For this review, take the finished solid that the model builds, in its own axes (mm). A direction names the side the tool comes from. Give positions to 0.01 mm unless a question says otherwise; leave off trailing zeros. Write each loop counter-clockwise with the first axis right and the second up, starting at its lowest first coordinate (ties: lowest second). Pieces come first, ordered by that corner, then holes. Notation, with made-up numbers: M 31,29.5 L 63,29.5 A25 cw 63,60.5 Z; hole C -20,70.25 d4. An arc over 180 degrees is marked long. One line per item, written item: value. Start each with the question number.
Item 1: Consider section B-B, the plane z = 4. Write out the cut boundary in (x, y) (3 decimals), and give its area (3 significant figures).
Item 2: Clearance check with a flat-ended pin moving along its axis: pin 1 Ø4.5 at (x, y) = (40, 106.825) entering from -Z. State where the tip first meets the part, or that it passes through.
Item 3: Mouldability with a two-part tool opening along Y and no side actions: class faces 1 (the face through (-40.26, 108.81, 3.13)), 2 (the face through (25, -77, 3)), 3 (the face through (-1, 2, 6.35)), 4 (the face through (-1, -110, 3)) as released by +Y, released by -Y, zero draft, split by the parting line, or undercut.
Item 4: Tool access review of faces 5 (the face through (-1, 2, 0)), 6 (the face through (-20, -47, 3)): name each direction out of +Z, -Z, +X, -X, +Y, -Y from which nothing blocks a thin tool from reaching the whole face with its end or side.
Item 5: Consider section A-A, the plane x = 40. Write out the cut boundary in (y, z) (3 decimals), and give its area (3 significant figures).
Item 6: Consider section C-C, the plane x = -20. Write out the cut boundary in (y, z), and give its area (3 significant figures).
Item 7: To check wall thickness, follow probe 1 along Y at (x, z) = (0, 2.25) (3 decimals); probe 2 along X at (y, z) = (-68, 4); probe 3 along Y at (x, z) = (20, 5.25). State the ranges of each line that lie inside material, in increasing order.
```python
from build123d import *

# Parameters (mm, degrees)
CROQUIS1_W              = 110
CROQUIS1_H              = 220
SALIENTE_EXTRUIR1_DEPTH = 6.35
CROQUIS2_R              = 2
CORTAR_EXTRUIR2_DEPTH   = 7.35


with BuildPart() as part:
    # Croquis1 → Saliente-Extruir1 (new body)
    with BuildSketch(Plane.XY):
        Rectangle(CROQUIS1_W, CROQUIS1_H)
    extrude(amount=SALIENTE_EXTRUIR1_DEPTH)

    # Croquis2 → Cortar-Extruir2 (cut, through all)
    with BuildSketch(Plane.XY):
        with Locations((40, 106.825)):
            Circle(CROQUIS2_R)
        with Locations((-40, 106.825)):
            Circle(CROQUIS2_R)
        with Locations((0, 106.825)):
            Circle(CROQUIS2_R)
        with BuildLine():
            Line((-25, -52), (-25, -102))
            ThreePointArc((-25, -102), (-20, -107), (-15, -102))
            Line((-15, -102), (-15, -52))
            ThreePointArc((-15, -52), (-20, -47), (-25, -52))
        make_face()
        with BuildLine():
            Line((15, -52), (15, -102))
            ThreePointArc((15, -102), (20, -107), (25, -102))
            Line((25, -102), (25, -52))
            ThreePointArc((25, -52), (20, -47), (15, -52))
        make_face()
    extrude(amount=CORTAR_EXTRUIR2_DEPTH, mode=Mode.SUBTRACT)


solid = part.part
```
Model answer:
1. outline: M -55,-110 L 55,-110 L 55,110 L -55,110 Z; hole C -40,106.825 d4; hole M -25,-102 A5 ccw -15,-102 L -15,-52 A5 ccw -25,-52 Z; hole C 0,106.825 d4; hole M 15,-102 A5 ccw 25,-102 L 25,-52 A5 ccw 15,-52 Z; hole C 40,106.825 d4
1. area: 23,000 mm2
2. pin 1: stops at z = 0
3. face 1: undercut
3. face 2: undercut
3. face 3: zero draft
3. face 4: released by -Y
4. face 5: -Z, +X, -X, +Y, -Y
4. face 6: +Z, -Z
5. outline: M -110,0 L 104.825,0 L 104.825,6.35 L -110,6.35 Z; M 108.825,0 L 110,0 L 110,6.35 L 108.825,6.35 Z
5. area: 1,370 mm2
6. outline: M -110,0 L -107,0 L -107,6.35 L -110,6.35 Z; M -47,0 L 110,0 L 110,6.35 L -47,6.35 Z
6. area: 1,020 mm2
7. probe 1: y = -110 to 104.825, 108.825 to 110
7. probe 2: x = -55 to -25, -15 to 15, 25 to 55
7. probe 3: y = -110 to -107, -47 to 110
